Autodesk Fusion 360 part; units mm, degrees
sketch "Sketch1" plane through (0, 0, 0) normal (0, 0, 1) x (1, 0, 0)
  line L0 (0, 0) -> (7.8, 0)
  line L1 (7.8, 0) -> (7.8, 31.8)
  line L2 (7.8, 31.8) -> (0, 31.8)
  line L3 (0, 31.8) -> (0, 0)
  dimension "d1" = 7.8
  dimension "d2" = 31.8
extrude "Extrude1" add sketch "Sketch1" along normal blind 3.1
sketch "Sketch2" plane through (0, 0, 0) normal (0, 0, -1) x (1, 0, 0)
  line L0 (0, 0) -> (0, -31.8)
  line L1 (0, -31.8) -> (7.8, -31.8)
  line L2 (7.8, -31.8) -> (7.8, 0)
  line L3 (7.8, 0) -> (0, 0)
  line L4 (1.4, -1.4) -> (6.4, -1.4)
  line L5 (6.4, -1.4) -> (6.4, -30.4)
  line L6 (6.4, -30.4) -> (1.4, -30.4)
  line L7 (1.4, -30.4) -> (1.4, -1.4)
  dimension "d5" = 1.4
  dimension "d6" = 1.4
  dimension "d7" = 1.4
  dimension "d8" = 1.4
extrude "Extrude2" cut sketch "Sketch2" against normal blind 2 contours L4 L5 L6 L7
sketch "Sketch3" plane through (0, 0, 3.1) normal (0, 0, 1) x (-1, 0, 0)
  line L0 (0, -31.8) -> (0, 0)
  line L1 (0, 0) -> (-7.8, 0)
  line L2 (-7.8, 0) -> (-7.8, -31.8)
  line L3 (-7.8, -31.8) -> (0, -31.8)
  circle A0 centre (-3.9, -27.825) radius 2.4
  circle A1 centre (-3.997, -19.875) radius 2.4
  circle A2 centre (-4.0941, -11.925) radius 2.4
  circle A3 centre (-4.1911, -3.975) radius 2.4
  dimension "d11" = 4.8
  dimension "d12" = 4.8
  dimension "d13" = 4.8
  dimension "d14" = 4.8
  dimension "d15" = 3.9
  dimension "d16" = 7.95
  dimension "d17" = 7.95
  dimension "d18" = 7.95
  dimension "d19" = 3.975
extrude "Extrude3" add sketch "Sketch3" along normal blind 1.6 contours A0 | A1 | A2 | A3
sketch "Sketch4" plane through (0, 0, 2) normal (0, 0, -1) x (1, 0, 0)
  line L0 (1.4, -30.4) -> (6.4, -30.4)
  line L1 (6.4, -30.4) -> (6.4, -1.4)
  line L2 (6.4, -1.4) -> (1.4, -1.4)
  line L3 (1.4, -1.4) -> (1.4, -30.4)
  circle A0 centre (3.9, -7.95) radius 1.45
  circle A1 centre (3.9, -15.9) radius 1.45
  circle A2 centre (3.9, -23.85) radius 1.45
  circle A3 centre (3.9, -7.95) radius 0.75
  circle A4 centre (3.9, -15.9) radius 0.75
  circle A5 centre (3.9, -23.85) radius 0.75
  dimension "d22" = 2.9
  dimension "d23" = 2.9
  dimension "d24" = 2.9
  dimension "d28" = 7.95
  dimension "d29" = 7.95
  dimension "d30" = 7.95
  dimension "d31" = 3.9
  dimension "d32" = 1.5
  dimension "d33" = 1.5
  dimension "d34" = 1.5
extrude "Extrude4" add sketch "Sketch4" along normal blind 2 contours A0 | A1 | A2
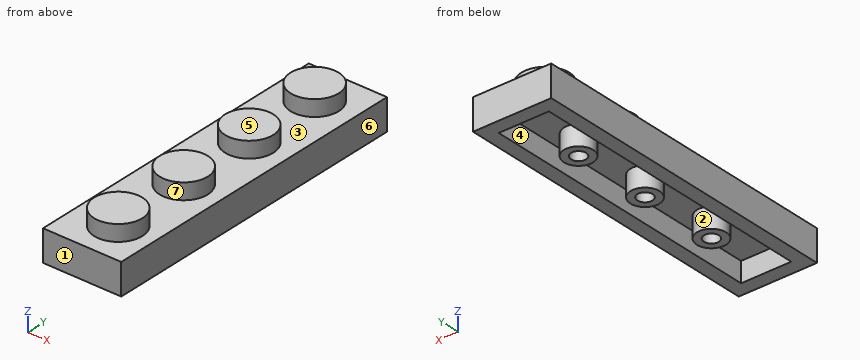
Work out the finished part from the listing and answer in its coordinate system (mm). Face numbers are marked on the shaded views. A direction names the side the tool comes from. Round coordinates to 2 decimals unless told otherwise and drop trailing zeros. Loops run counter-clockwise (first coordinate to the right, second up) from the corner with the lowest first, then second, coordinate; pieces in that order, holes last. Notation, with made-up numbers: M -38.75,31.5 L 14.25,31.5 A19 ccw 14.25,58.5 Z; hole C -5.5,39.25 d8. An arc over 180 degrees is marked long. Use CSV: the item, a comma, the result in double quotes.
Q1. A tool of negligible diameter and unlimited length cuts with its end or side. For the marked faces 1, 2 and 3, from which of +Z, -Z, +X, -X, +Y, -Y can it reach the whole face along a straight path? Write none if from no direction.
Determined:
face 1,"+Z, -Z, +X, -X, -Y"
face 2,"-Z"
face 3,"+Z"
Q2. Consider L1, parallel to X at y = 7.95, z = 0.95; L2, parallel to Y at x = 5.75, z = 1.6; L3, parallel to X at y = 5, z = 0.35. Determine where each line is inside the solid, lowest interval first.
Determined:
L1,"0 to 1.4, 2.45 to 3.15, 4.65 to 5.35, 6.4 to 7.8"
L2,"0 to 1.4, 30.4 to 31.8"
L3,"0 to 1.4, 6.4 to 7.8"
Q3. Section C-C, the plane z = 3.9 is taken. Determine the outline of the cut face in (x, y) (3 decimals).
Determined:
outline,"C 3.9,27.825 d4.8; C 3.997,19.875 d4.8; C 4.094,11.925 d4.8; C 4.191,3.975 d4.8"
Q4. Each of these flat-tipped pins is pushed along its axis until it touches: pin 1 (2 mm diameter, centred on x = 5, y = 11, fed in from -Z); pin 2 (1.6 mm diameter, centred on x = 4, y = 23.5, fed in from -Z); pin 3 (1.5 mm diameter, centred on y = 19.5, z = 4, fed in from +X); pin 4 (1 mm diameter, centred on x = 4, y = 24, fed in from +Z). Where does it stop, or does it pass through?
Determined:
pin 1,"z = 2"
pin 2,"z = 0"
pin 3,"x = 6.4"
pin 4,"z = 3.1"
Q5. Section B-B, the plane y = 7.95 is taken. Determine the outline of the cut face in (x, z).
Determined:
outline,"M 0,0 L 1.4,0 L 1.4,2 L 2.45,2 L 2.45,0 L 3.15,0 L 3.15,2 L 4.65,2 L 4.65,0 L 5.35,0 L 5.35,2 L 6.4,2 L 6.4,0 L 7.8,0 L 7.8,3.1 L 0,3.1 Z"
Q6. The mould has two halves that part along X. Classify the marked faces 4, 5, 6 and 7: pulls with the +X half, pulls with the -X half, needs draft (parallel to the pull), parting line crosses it, or undercut.
Determined:
face 4,"undercut"
face 5,"needs draft"
face 6,"pulls with the +X half"
face 7,"parting line crosses it"
Q7. Section A-A, the plane z = 1.7 is taken. Determine the outline of the cut face in (x, y), then the cut area to 3 significant figures.
Determined:
outline,"M 0,0 L 7.8,0 L 7.8,31.8 L 0,31.8 Z; C 3.9,7.95 d2.9; C 3.9,15.9 d2.9; C 3.9,23.85 d2.9; hole M 1.4,1.4 L 6.4,1.4 L 6.4,30.4 L 1.4,30.4 Z; hole C 3.9,7.95 d1.5; hole C 3.9,15.9 d1.5; hole C 3.9,23.85 d1.5"
area,"118 mm2"
